Input: part model. Units: mm. Frame: model coordinates. Face numbers are marked on the shaded views. A direction names the side the tool comes from. Round coordinates to 2 decimals unless told otherwise and drop trailing zeros. Write each loop counter-clockwise with the first axis right and the second up, starting at its lowest first coordinate (ties: lowest second). Pieces come first, ordered by that corner, then holes. Notation, with made-up numbers: (52, 89.5) -> (63, 89.5) arc R25 ccw to (63, 103.5) -> close; hole circle Ø6 at (49.25, 84.25). An arc over 180 degrees is marked (long way). Write item = value, one per line.
```python
from build123d import *

# Parameters (mm, degrees)
SKETCH1_W                                           = 14
SKETCH1_H                                           = 77
BOSS_EXTRUDE1_DEPTH                                 = 3.5
CBORE_FOR_M3_HEX_SOCKET_HEAD_CAP_SCREW1_D           = 3.2
CBORE_FOR_M3_HEX_SOCKET_HEAD_CAP_SCREW1_CBORE_D     = 6.5
CBORE_FOR_M3_HEX_SOCKET_HEAD_CAP_SCREW1_CBORE_DEPTH = 3.4
SKETCH4_R                                           = 3.5
CUT_EXTRUDE1_DEPTH                                  = 40.752358421
FILLET1_R                                           = 1
FILLET2_R                                           = 1


with BuildPart() as part:
    # Sketch1 → Boss-Extrude1 (new, symmetric)
    with BuildSketch(Plane.XY):
        Rectangle(SKETCH1_W, SKETCH1_H)
    extrude(amount=BOSS_EXTRUDE1_DEPTH, both=True)

    # CBORE for M3 Hex Socket Head Cap Screw1 (through all)
    with Locations(Plane.XY.offset(3.5)):
        with Locations((0, -30), (0, 30)):
            CounterBoreHole(CBORE_FOR_M3_HEX_SOCKET_HEAD_CAP_SCREW1_D / 2, CBORE_FOR_M3_HEX_SOCKET_HEAD_CAP_SCREW1_CBORE_D / 2, CBORE_FOR_M3_HEX_SOCKET_HEAD_CAP_SCREW1_CBORE_DEPTH)

    # Sketch4 → Cut-Extrude1 (cut, through all)
    with BuildSketch(Plane.XY.offset(3.5)):
        with Locations((0, -12.75)):
            Circle(SKETCH4_R)
        with Locations(Location((0, 12.75, 0), (0, 0, 180))):
            Circle(SKETCH4_R)
    extrude(amount=-CUT_EXTRUDE1_DEPTH, mode=Mode.SUBTRACT)

    # Fillet1
    fillet1_edges = [part.edges().sort_by_distance(p)[0] for p in [
        (-7, 38.5, 0),
        (7, 38.5, 0),
        (7, -38.5, 0),
        (-7, -38.5, 0),
    ]]
    fillet(fillet1_edges, radius=FILLET1_R)

    # Fillet2
    fillet2_edges = [part.edges().sort_by_distance(p)[0] for p in [
        (-7, 0, -3.5),
        (-7, 0, 3.5),
        (0, 38.5, -3.5),
        (7, 0, -3.5),
        (0, -38.5, -3.5),
        (6.707106781, 38.207106781, -3.5),
        (6.707106781, -38.207106781, -3.5),
        (-6.707106781, -38.207106781, -3.5),
        (-6.707106781, 38.207106781, -3.5),
        (0, 38.5, 3.5),
        (0, -38.5, 3.5),
        (7, 0, 3.5),
        (6.707106781, 38.207106781, 3.5),
        (6.707106781, -38.207106781, 3.5),
        (-6.707106781, -38.207106781, 3.5),
        (-6.707106781, 38.207106781, 3.5),
    ]]
    fillet(fillet2_edges, radius=FILLET2_R)


solid = part.part
```
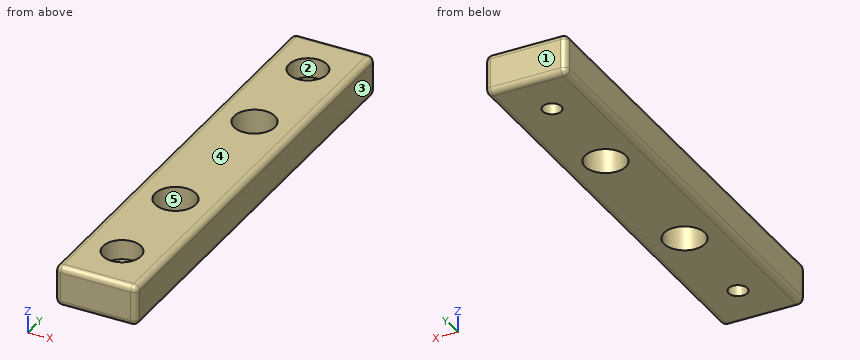
1) Cut plane B-B (z = -1.5). Return the cut outline in (x, y).
Solutions:
outline = (-7, -37.5) arc R1 ccw to (-6, -38.5) -> (6, -38.5) arc R1 ccw to (7, -37.5) -> (7, 37.5) arc R1 ccw to (6, 38.5) -> (-6, 38.5) arc R1 ccw to (-7, 37.5) -> close; hole circle Ø7 at (0, -12.75); hole circle Ø7 at (0, 12.75); hole circle Ø3.2 at (0, -30); hole circle Ø3.2 at (0, 30)
2) Cut plane D-D (y = 12.75). Return the cut outline in (x, z), and give its area (3 significant figures).
Solutions:
outline = (-7, -2.5) arc R1 ccw to (-6, -3.5) -> (-3.5, -3.5) -> (-3.5, 3.5) -> (-6, 3.5) arc R1 ccw to (-7, 2.5) -> close; (3.5, -3.5) -> (6, -3.5) arc R1 ccw to (7, -2.5) -> (7, 2.5) arc R1 ccw to (6, 3.5) -> (3.5, 3.5) -> close
area = 48.1 mm^2
3) Line query: L1, parallel to Y at x = 0, z = 1.05; L2, parallel to Y at x = 0, z = -2; L3, parallel to X at y = -12.5, z = 1.75. Output: solid intervals per line, ascending. Write a range as from..to.
Solutions:
L1 = -38.5..-33.25, -26.75..-16.25, -9.25..9.25, 16.25..26.75, 33.25..38.5
L2 = -38.5..-31.6, -28.4..-16.25, -9.25..9.25, 16.25..28.4, 31.6..38.5
L3 = -7..-3.49, 3.49..7
4) Cut plane A-A (y = 30). Return the cut outline in (x, z), and give its area (3 significant figures).
Solutions:
outline = (-7, -2.5) arc R1 ccw to (-6, -3.5) -> (-1.6, -3.5) -> (-1.6, 0.1) -> (-3.25, 0.1) -> (-3.25, 3.5) -> (-6, 3.5) arc R1 ccw to (-7, 2.5) -> close; (1.6, -3.5) -> (6, -3.5) arc R1 ccw to (7, -2.5) -> (7, 2.5) arc R1 ccw to (6, 3.5) -> (3.25, 3.5) -> (3.25, 0.1) -> (1.6, 0.1) -> close
area = 63.5 mm^2
5) Access query for the marked faces 1 and 2. Directions: +Z, -Z, +X, -X, +Y, -Y. A direction counts if a zero-diameter tool reaches every point of the face in a straight line with its end or side. Return the directions, or none.
Solutions:
face_1 = +Z, -Z, +X, -X, +Y
face_2 = +Z
6) Cut plane C-C (x = 0). Count the separate pieces of the cut face and the enclosed holes in it, and give its area (3 significant figures).
Solutions:
separate_pieces = 5
enclosed_holes = 0
area = 373 mm^2
7) First-contact query: P1, Ø3.5, axis at x = 0, y = 30, coming from the +Z side; P2, Ø3, axis at x = 0, y = -30, coming from the -Z side. Flat tips, straight axial feed; report the tip coordinate or a pass-through.
Solutions:
P1 = 0.1
P2 = through
8) Draft query along X for the marked faces 3, 4 and 5. Return one class per face: +X half, -X half, draft (parallel to the pull), parting line (faces both ways), or undercut.
Solutions:
face_3 = +X half
face_4 = draft
face_5 = undercut
